Geometry: final body of the model. Coordinates: model frame, mm. A direction names the side the tool comes from. Give positions to 0.01 mm unless a question says otherwise; leave off trailing zeros. Write each loop counter-clockwise with the first axis right and the second up, starting at its lowest first coordinate (ties: lowest second). Pieces come first, ordered by that corner, then holes. Notation, with made-up numbers: (53, 55) - (96, 55) arc R34 cw to (96, 90) - close; hole circle Ø11 at (15, 20). An arc over 180 degrees is marked (long way). Return JSON: item names as keys, results as strings.
from build123d import *

# Parameters (mm, degrees)
F1_DEPTH = 25.4
F3_DEPTH = 34.544


with BuildPart() as f1:
    # F0 (on Top) → F1 (new body)
    with BuildSketch(Plane.XY):
        with BuildLine():
            Line((-70.7662329078, 55.5032007331), (-70.7662329078, 6.4394138818))
            ThreePointArc((-70.7662329078, 6.4394138818), (-37.7403006525, 2.8219468482), (-20.0934376224, 30.9713073075))
            ThreePointArc((-20.0934376224, 30.9713073075), (-37.7403006525, 59.1206677668), (-70.7662329078, 55.5032007331))
        make_face()
        with BuildLine():
            ThreePointArc((-70.7662329078, 55.5032007331), (-82.6427001849, 30.9713073075), (-70.7662329078, 6.4394138818))
            Line((-70.7662329078, 6.4394138818), (-70.7662329078, 55.5032007331))
        make_face()
    extrude(amount=F1_DEPTH)

    # F2 (on face) → F3 (join)
    with BuildSketch(Plane.XY.offset(25.4)):
        Polygon((-63.1933323456, 10.1122700805), (-47.8355326341, 17.3510151719), (-46.425569919, 34.2706324141), (-60.3734069155, 43.9515045648), (-75.7312066271, 36.7127594734), (-77.1411693421, 19.7931422312), align=None)
    extrude(amount=F3_DEPTH)


solid = f1.part
Q1. Section query A-A, the plane z = 29.5. Return the cut outline in (x, y).
Answer key:
{"outline": "(-77.14, 19.79) - (-63.19, 10.11) - (-47.84, 17.35) - (-46.43, 34.27) - (-60.37, 43.95) - (-75.73, 36.71) - close"}
Q2. Section query D-D, the plane z = 18. Return the cut outline in (x, y), plus the area to 3 significant figures.
Answer key:
{"outline": "circle Ø62.55 at (-51.37, 30.97)", "area": "3,070 mm^2"}
Q3. Pin query (flat end, axial travel): P1, Ø12, axis at x = -30.5, z = 23.5, coming from the +Y side; P2, Ø10, axis at x = -48.5, z = 34, coming from the +Y side; P3, Ø8, axis at x = -60.5, y = 25.5, coming from the -Z side; P4, Ø12, axis at x = -44, z = 22.5, coming from the +Y side. Return the tip coordinate at first contact, or that it passes through.
Answer key:
{"P1": "stops at y = 58.49", "P2": "stops at y = 39.18", "P3": "stops at z = 0", "P4": "stops at y = 62.22"}
Q4. Section query B-B, the plane y = 15.5. Return the cut outline in (x, z).
Answer key:
{"outline": "(-78.55, 0) - (-24.19, 0) - (-24.19, 25.4) - (-51.76, 25.4) - (-51.76, 59.94) - (-70.96, 59.94) - (-70.96, 25.4) - (-78.55, 25.4) - close"}
Q5. Section query C-C, the plane x = -59. Return the cut outline in (y, z).
Answer key:
{"outline": "(0.64, 0) - (61.3, 0) - (61.3, 25.4) - (43, 25.4) - (43, 59.94) - (12.09, 59.94) - (12.09, 25.4) - (0.64, 25.4) - close"}
Q6. Material intervals for probe 1 along Z at (x, y) = (-46, 7); probe 2 along X at (y, z) = (31.5, 16); probe 3 along Y at (x, z) = (-51, 15.5), sorted ascending. Write a range as [from, to].
Answer key:
{"probe 1": "z = [0, 25.4]", "probe 2": "x = [-82.64, -20.1]", "probe 3": "y = [-0.3, 62.24]"}
Q7. Set-up query: faces 1 (the flat face through (-53.3, 39.04, 42.43)), 2 (the flat face through (-47.14, 25.69, 42.43)), 3 (the flat face through (-67.945, 40.383, 42.43)), 4 (the flat face through (-70.265, 15.02, 42.43)). Return all of +Z, -Z, +X, -X, +Y, -Y with unobstructed straight access to the full face (end or side cutting, diameter ignored); none if empty.
Answer key:
{"face 1": "+Z, +X, +Y", "face 2": "+Z, +X, -Y", "face 3": "+Z, -X, +Y", "face 4": "+Z, -X, -Y"}
